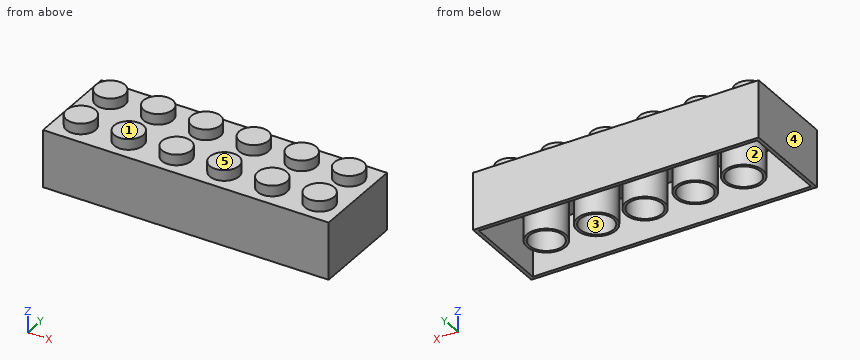
from build123d import *

# Parameters (mm, degrees)
F0_W      = 47.7774
F0_H      = 15.8369
F1_DEPTH  = 4.7879
F2_R      = 2.4511
F14_DEPTH = 1.778
F3_R      = 2.4511
F15_DEPTH = 1.778
F4_R      = 2.4511
F16_DEPTH = 1.778
F5_R      = 2.4511
F17_DEPTH = 1.778
F6_R      = 2.4511
F18_DEPTH = 1.778
F7_R      = 2.4511
F19_DEPTH = 1.778
F8_R      = 2.4511
F20_DEPTH = 1.778
F9_R      = 2.4511
F21_DEPTH = 1.778
F10_R     = 2.4511
F22_DEPTH = 1.778
F11_R     = 2.4511
F23_DEPTH = 1.778
F12_R     = 2.4511
F24_DEPTH = 1.778
F13_R     = 2.4511
F25_DEPTH = 1.778
F30_W     = 46.5582
F30_H     = 14.6304
F30_R     = 3.2385
F37_DEPTH = 8.3312
F27_R     = 3.2385
F38_DEPTH = 8.3312
F32_R     = 2.794
F39_DEPTH = 8.3312
F28_R     = 3.2385
F40_DEPTH = 8.3312
F29_R     = 3.2385
F41_DEPTH = 8.3312
F31_R     = 3.2385
F42_DEPTH = 8.3312
F33_R     = 2.794
F43_DEPTH = 8.3312
F34_R     = 2.794
F44_DEPTH = 8.3312
F35_R     = 2.794
F45_DEPTH = 8.3312
F36_R     = 2.794
F46_DEPTH = 8.3312


with BuildPart() as f1:
    # F0 (on Top) → F1 (new body, symmetric)
    with BuildSketch(Plane.XY):
        Rectangle(F0_W, F0_H)
    extrude(amount=F1_DEPTH, both=True)

    # F2 (on face) → F14 (join)
    with BuildSketch(Plane.XY.offset(4.7879)):
        with Locations((-19.9644, 3.99415)):
            Circle(F2_R)
    extrude(amount=F14_DEPTH)

    # F3 (on face) → F15 (join)
    with BuildSketch(Plane.XY.offset(4.7879)):
        with Locations((-11.9634, 3.99415)):
            Circle(F3_R)
    extrude(amount=F15_DEPTH)

    # F4 (on face) → F16 (join)
    with BuildSketch(Plane.XY.offset(4.7879)):
        with Locations((-3.9624, 3.99415)):
            Circle(F4_R)
    extrude(amount=F16_DEPTH)

    # F5 (on face) → F17 (join)
    with BuildSketch(Plane.XY.offset(4.7879)):
        with Locations((4.0386, 3.99415)):
            Circle(F5_R)
    extrude(amount=F17_DEPTH)

    # F6 (on face) → F18 (join)
    with BuildSketch(Plane.XY.offset(4.7879)):
        with Locations((12.0396, 3.99415)):
            Circle(F6_R)
    extrude(amount=F18_DEPTH)

    # F7 (on face) → F19 (join)
    with BuildSketch(Plane.XY.offset(4.7879)):
        with Locations((19.9644, 3.99415)):
            Circle(F7_R)
    extrude(amount=F19_DEPTH)

    # F8 (on face) → F20 (join)
    with BuildSketch(Plane.XY.offset(4.7879)):
        with Locations((-19.9644, -3.99415)):
            Circle(F8_R)
    extrude(amount=F20_DEPTH)

    # F9 (on face) → F21 (join)
    with BuildSketch(Plane.XY.offset(4.7879)):
        with Locations((-11.9634, -3.99415)):
            Circle(F9_R)
    extrude(amount=F21_DEPTH)

    # F10 (on face) → F22 (join)
    with BuildSketch(Plane.XY.offset(4.7879)):
        with Locations((-3.9624, -3.99415)):
            Circle(F10_R)
    extrude(amount=F22_DEPTH)

    # F11 (on face) → F23 (join)
    with BuildSketch(Plane.XY.offset(4.7879)):
        with Locations((4.0386, -3.99415)):
            Circle(F11_R)
    extrude(amount=F23_DEPTH)

    # F12 (on face) → F24 (join)
    with BuildSketch(Plane.XY.offset(4.7879)):
        with Locations((12.0396, -3.99415)):
            Circle(F12_R)
    extrude(amount=F24_DEPTH)

    # F13 (on face) → F25 (join)
    with BuildSketch(Plane.XY.offset(4.7879)):
        with Locations((19.9644, -3.99415)):
            Circle(F13_R)
    extrude(amount=F25_DEPTH)

    # F30 (on face) → F37 (cut)
    with BuildSketch(Plane(origin=(0, 0, -4.7879), x_dir=(1, 0, 0), z_dir=(0, 0, -1))):
        Rectangle(F30_W, F30_H)
        with Locations((8.1026, 0)):
            Circle(F30_R, mode=Mode.SUBTRACT)
    extrude(amount=-F37_DEPTH, mode=Mode.SUBTRACT)

    # F27 (on face) → F38 (join)
    with BuildSketch(Plane(origin=(0, 0, -4.7879), x_dir=(1, 0, 0), z_dir=(0, 0, -1))):
        with Locations((-16.51, 0)):
            Circle(F27_R)
    extrude(amount=-F38_DEPTH)

    # F32 (on face) → F39 (cut)
    with BuildSketch(Plane(origin=(0, 0, -4.7879), x_dir=(1, 0, 0), z_dir=(0, 0, -1))):
        with Locations((-16.491707, 0)):
            Circle(F32_R)
    extrude(amount=-F39_DEPTH, mode=Mode.SUBTRACT)

    # F28 (on face) → F40 (join)
    with BuildSketch(Plane(origin=(0, 0, -4.7879), x_dir=(1, 0, 0), z_dir=(0, 0, -1))):
        with Locations((-8.4074, 0)):
            Circle(F28_R)
    extrude(amount=-F40_DEPTH)

    # F29 (on face) → F41 (join)
    with BuildSketch(Plane(origin=(0, 0, -4.7879), x_dir=(1, 0, 0), z_dir=(0, 0, -1))):
        Circle(F29_R)
    extrude(amount=-F41_DEPTH)

    # F31 (on face) → F42 (join)
    with BuildSketch(Plane(origin=(0, 0, -4.7879), x_dir=(1, 0, 0), z_dir=(0, 0, -1))):
        with Locations((16.51, 0)):
            Circle(F31_R)
    extrude(amount=-F42_DEPTH)

    # F33 (on face) → F43 (cut)
    with BuildSketch(Plane(origin=(0, 0, -4.7879), x_dir=(1, 0, 0), z_dir=(0, 0, -1))):
        with Locations((-8.388528, 0)):
            Circle(F33_R)
    extrude(amount=-F43_DEPTH, mode=Mode.SUBTRACT)

    # F34 (on face) → F44 (cut)
    with BuildSketch(Plane(origin=(0, 0, -4.7879), x_dir=(1, 0, 0), z_dir=(0, 0, -1))):
        Circle(F34_R)
    extrude(amount=-F44_DEPTH, mode=Mode.SUBTRACT)

    # F35 (on face) → F45 (cut)
    with BuildSketch(Plane(origin=(0, 0, -4.7879), x_dir=(1, 0, 0), z_dir=(0, 0, -1))):
        with Locations((8.077325, 0)):
            Circle(F35_R)
    extrude(amount=-F45_DEPTH, mode=Mode.SUBTRACT)

    # F36 (on face) → F46 (cut)
    with BuildSketch(Plane(origin=(0, 0, -4.7879), x_dir=(1, 0, 0), z_dir=(0, 0, -1))):
        with Locations((16.506594, 0)):
            Circle(F36_R)
    extrude(amount=-F46_DEPTH, mode=Mode.SUBTRACT)


solid = f1.part
Design review of the part built by this model. Coordinates are the model's own, in mm. Face numbers are marked on the shaded views. A direction names the side the tool comes from. Give positions to 0.01 mm unless a question says otherwise; leave off trailing zeros. Write each loop counter-clockwise with the first axis right and the second up, starting at its lowest first coordinate (ties: lowest second). Pieces come first, ordered by that corner, then holes. Notation, with made-up numbers: M 32,71 L 43,71 A17 cw 43,93 Z; hole C 17,-38 d7. An arc over 180 degrees is marked long. Answer as a JSON object with one key per item and string values. Group by question number.
1) For line 1 along Y through (x, z) = (-17.5, 0.5); line 2 along Y through (x, z) = (10, 0); line 3 along X through (y, z) = (-3.5, -3.25), list the stretches that pass through material, from the lowest coordinate up.
2) Tool access review of the marked faces 1 and 2: name each direction out of +Z, -Z, +X, -X, +Y, -Y from which nothing blocks a thin tool from reaching the whole face with its end or side.
3) We need section B-B (x = 16.51). Give the boundary of the cut face in (y, z), and give its area (3 significant figures).
4) We need section A-A (z = 2.75). Count the separate pieces of the cut face and the enclosed holes in it, and give its area (3 significant figures).
5) Mouldability with a two-part tool opening along X and no side actions: class the marked faces 3, 4 and 5 as released by +X, released by -X, zero draft, split by the parting line, or undercut.
6) Clearance check with flat-ended pins moving along their axes: pin 1 Ø3.5 at (x, y) = (8.08, 0) entering from +Z; pin 2 Ø1.7 at (x, y) = (17.5, -1.5) entering from -Z. State where each tip first meets the part, or that it passes through.
Answer key:
{
 "1": {"line 1": "y = -7.92 to -7.32, -3.08 to -2.61, 2.61 to 3.08, 7.32 to 7.92", "line 2": "y = -7.92 to -7.32, -2.62 to -2.03, 2.03 to 2.62, 7.32 to 7.92", "line 3": "x = -23.89 to -23.28, 23.28 to 23.89"},
 "2": {"face 1": "+Z, +X, -X, +Y, -Y", "face 2": "-Z"},
 "3": {"outline": "M -7.92,-4.79 L -7.32,-4.79 L -7.32,3.54 L -3.24,3.54 L -3.24,-4.79 L -2.79,-4.79 L -2.79,3.54 L 2.79,3.54 L 2.79,-4.79 L 3.24,-4.79 L 3.24,3.54 L 7.32,3.54 L 7.32,-4.79 L 7.92,-4.79 L 7.92,4.79 L -7.92,4.79 Z", "area": "37.2 mm²"},
 "4": {"separate pieces": "6", "enclosed holes": "6", "area": "118 mm²"},
 "5": {"face 3": "undercut", "face 4": "released by -X", "face 5": "zero draft"},
 "6": {"pin 1": "stops at z = 4.79", "pin 2": "stops at z = 3.54"}
}
